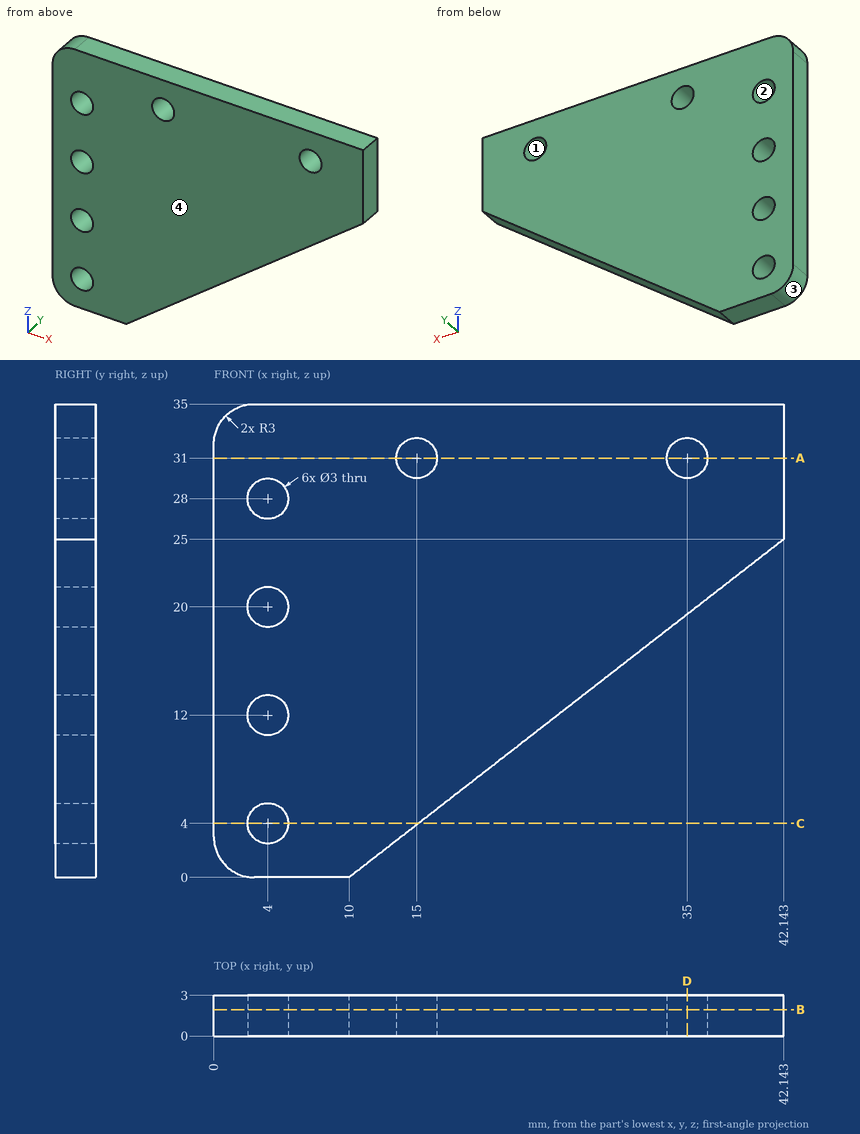
Study the drawing (mm; zero at the part's minimum x, y, z) and answer. Give positions to 0.01 mm unless a question says otherwise; leave off trailing zeros. Write each loop counter-clockwise with the first axis right and the second up, starting at its lowest first coordinate (ties: lowest second). Pieces come first, ordered by that corner, then holes. Notation, with made-up numbers: (5, 46) - (21, 46) arc R25 ccw to (21, 76) - close; hole circle Ø9 at (54.5, -1). An arc over 180 degrees is marked (long way). Use CSV: the item, a comma, the result in double quotes. Start each with the question number.
(1) Given P1, Ø4, axis at x = 4, z = 28, coming from the -Y side; P2, Ø1, axis at x = 30, y = 1.5, coming from the -Z side, each flat-ended and moving along its own axis, determine where each tip first touches the part or whether it passes through.
(2) Find section C-C (z = 4). Give the vertices of the cut face in (x, y).
(3) Determine the mould class of the marked faces 1, 2, 3 and 4 for opening direction Z: +Z half, -Z half, draft (parallel to the pull), parting line (faces both ways), or undercut.
(4) Consider line 1 along X through (y, z) = (2.1, 31); line 2 along X through (y, z) = (0.65, 12); line 3 along X through (y, z) = (0.95, 4). Determine where each line is inside the solid, lowest interval first.
(5) Find section B-B (y = 1.95). Give the vertices of the cut face in (x, z).
(6) Find section D-D (x = 35). Give the vertices of the cut face in (y, z).
(7) Find section A-A (z = 31). Give the vertices of the cut face in (x, y).
Findings below:
1,P1,"y = 0"
1,P2,"z = 15.17"
2,outline,"(0, 0) - (2.5, 0) - (2.5, 3) - (0, 3) - close; (5.5, 0) - (15.14, 0) - (15.14, 3) - (5.5, 3) - close"
3,face 1,"undercut"
3,face 2,"undercut"
3,face 3,"-Z half"
3,face 4,"draft"
4,line 1,"0 to 13.5, 16.5 to 33.5, 36.5 to 42.14"
4,line 2,"0 to 2.5, 5.5 to 25.43"
4,line 3,"0 to 2.5, 5.5 to 15.14"
5,outline,"(0, 3) arc R3 ccw to (3, 0) - (10, 0) - (42.14, 25) - (42.14, 35) - (3, 35) arc R3 ccw to (0, 32) - close; hole circle Ø3 at (4, 4); hole circle Ø3 at (4, 12); hole circle Ø3 at (4, 20); hole circle Ø3 at (4, 28); hole circle Ø3 at (15, 31); hole circle Ø3 at (35, 31)"
6,outline,"(0, 19.44) - (3, 19.44) - (3, 29.5) - (0, 29.5) - close; (0, 32.5) - (3, 32.5) - (3, 35) - (0, 35) - close"
7,outline,"(0, 0) - (13.5, 0) - (13.5, 3) - (0, 3) - close; (16.5, 0) - (33.5, 0) - (33.5, 3) - (16.5, 3) - close; (36.5, 0) - (42.14, 0) - (42.14, 3) - (36.5, 3) - close"
